```python
from build123d import *

# Parameters (mm, degrees)
EXTRUDE_2_DEPTH     = 120
SKETCH_3_W          = 40
SKETCH_3_H          = 20.78460969
EXTRUDE_3_DEPTH     = 2
SKETCH_4_W          = 17.320508076
SKETCH_4_H          = 20.78460969
EXTRUDE_4_DEPTH     = 30
SKETCH_5_W          = 40
SKETCH_5_H          = 17.320508076
EXTRUDE_5_DEPTH     = 80
SKETCH_6_R          = 1.75
CUT_EXTRUDE_1_DEPTH = 234.786227139
SKETCH_7_R          = 3.25
CUT_EXTRUDE_2_DEPTH = 3.5
SKETCH_8_W          = 40
SKETCH_8_H          = 20
CUT_EXTRUDE_3_DEPTH = 1
SKETCH_10_W         = 40
SKETCH_10_H         = 20
CUT_EXTRUDE_4_DEPTH = 1
SKETCH_11_W         = 20
SKETCH_11_H         = 40
CUT_EXTRUDE_5_DEPTH = 1


with BuildPart() as part:
    # ｽｹｯﾁ2 → ﾎﾞｽ - 押し出し2 (new body)
    with BuildSketch(Plane(origin=(0, 0, 0), x_dir=(-1, 0, 0), z_dir=(0, 0, -1))):
        Polygon((12, -10.392304845), (0, 10.392304845), (-12, -10.392304845), align=None)
    extrude(amount=EXTRUDE_2_DEPTH)

    # ｽｹｯﾁ3 → ﾎﾞｽ - 押し出し3 (add)
    with BuildSketch(Plane(origin=(0, 0, -120), x_dir=(-1, 0, 0), z_dir=(0, 0, -1))):
        Rectangle(SKETCH_3_W, SKETCH_3_H)
    extrude(amount=EXTRUDE_3_DEPTH)

    # ｽｹｯﾁ4 → ﾎﾞｽ - 押し出し4 (add)
    with BuildSketch(Plane(origin=(0, 0, -122), x_dir=(-1, 0, 0), z_dir=(0, 0, -1))):
        Rectangle(SKETCH_4_W, SKETCH_4_H)
    extrude(amount=EXTRUDE_4_DEPTH)

    # ｽｹｯﾁ5 → ﾎﾞｽ - 押し出し5 (add)
    with BuildSketch(Plane(origin=(0, 0, -152), x_dir=(-1, 0, 0), z_dir=(0, 0, -1))):
        Rectangle(SKETCH_5_W, SKETCH_5_H)
    extrude(amount=EXTRUDE_5_DEPTH)

    # ｽｹｯﾁ6 → ｶｯﾄ - 押し出し1 (cut, through all)
    with BuildSketch(Plane(origin=(0, 10.392304845, 0), x_dir=(1, 0, 0), z_dir=(0, 1, 0))):
        with Locations(Location((-10, 162, 0), (0, 0, 270))):
            Circle(SKETCH_6_R)
        with Locations(Location((10, 162, 0), (0, 0, 270))):
            Circle(SKETCH_6_R)
        with Locations(Location((-10, 222, 0), (0, 0, 270))):
            Circle(SKETCH_6_R)
        with Locations(Location((10, 222, 0), (0, 0, 270))):
            Circle(SKETCH_6_R)
    extrude(amount=-CUT_EXTRUDE_1_DEPTH, mode=Mode.SUBTRACT)

    # ｽｹｯﾁ7 → ｶｯﾄ - 押し出し2 (cut)
    with BuildSketch(Plane(origin=(0, 10.392304845, 0), x_dir=(1, 0, 0), z_dir=(0, 1, 0))):
        with Locations(Location((-10, 162, 0), (0, 0, 270))):
            Circle(SKETCH_7_R)
        with Locations(Location((-10, 222, 0), (0, 0, 270))):
            Circle(SKETCH_7_R)
        with Locations(Location((10, 222, 0), (0, 0, 270))):
            Circle(SKETCH_7_R)
        with Locations(Location((10, 162, 0), (0, 0, 270))):
            Circle(SKETCH_7_R)
    extrude(amount=-CUT_EXTRUDE_2_DEPTH, mode=Mode.SUBTRACT)

    # ｽｹｯﾁ8 → ｶｯﾄ - 押し出し3 (cut)
    with BuildSketch(Plane(origin=(-4.5, 2.598076211, 0), x_dir=(0, 0, 1), z_dir=(-0.8660254037844386, 0.5000000000000001, 0))):
        with Locations((-95, -3)):
            Rectangle(SKETCH_8_W, SKETCH_8_H)
        with Locations((-25, -3)):
            Rectangle(SKETCH_8_W, SKETCH_8_H)
    extrude(amount=-CUT_EXTRUDE_3_DEPTH, mode=Mode.SUBTRACT)

    # ｽｹｯﾁ10 → ｶｯﾄ - 押し出し4 (cut)
    with BuildSketch(Plane(origin=(4.5, 2.598076211, 0), x_dir=(0, 0, -1), z_dir=(0.8660254037844387, 0.5000000000000001, 0))):
        with Locations((25, -3)):
            Rectangle(SKETCH_10_W, SKETCH_10_H)
        with Locations((95, -3)):
            Rectangle(SKETCH_10_W, SKETCH_10_H)
    extrude(amount=-CUT_EXTRUDE_4_DEPTH, mode=Mode.SUBTRACT)

    # ｽｹｯﾁ11 → ｶｯﾄ - 押し出し5 (cut)
    with BuildSketch(Plane(origin=(0, -10.392304845, 0), x_dir=(-1, 0, 0), z_dir=(0, -1, 0))):
        with Locations((0, 25)):
            Rectangle(SKETCH_11_W, SKETCH_11_H)
        with Locations((0, 95)):
            Rectangle(SKETCH_11_W, SKETCH_11_H)
    extrude(amount=-CUT_EXTRUDE_5_DEPTH, mode=Mode.SUBTRACT)


solid = part.part
```
For this review, take the finished solid that the model builds, in its own axes (mm). A direction names the side the tool comes from. Round coordinates to 2 decimals unless told otherwise and drop trailing zeros. Write each loop counter-clockwise with the first axis right and the second up, starting at its lowest first coordinate (ties: lowest second). Pieces come first, ordered by that corner, then holes. Notation, with made-up numbers: (87, 28) -> (119, 28) arc R12 ccw to (119, 42) -> close; hole circle Ø6 at (75, -34.5). An arc over 180 degrees is marked (long way). One line per question, with ' | ' between items. Start each with the question number.
(1) Add section C-C, the plane y = -1.25. Give the number of separate pieces and of enclosed holes in the cut face, plus the area to 3 significant figures.
(2) For line 1 along X through (y, z) = (8.05, -222); line 2 along Z through (x, y) = (-11.5, 5); line 3 along Z through (x, y) = (-7.5, -3), list the stretches that pass through material, from the lowest coordinate up. Write a range as from..to.
(3) Add section D-D, the plane z = -206.5. Write out the cut boundary in (x, y), plus the area to 3 significant figures.
(4) Insertion check: P1, Ø4, axis at x = 3, z = -176.5, coming from the -Y side; P2, Ø0.5, axis at y = -10, z = -31.5, coming from the +X side; P3, Ø3, axis at x = 9, z = -160.5, coming from the +Y side. Each pin has a flat end and moves straight along its axis. Give the tip position at first contact, or say it passes through.
(5) Add section A-A, the plane x = 17. Write out the cut boundary in (y, z), plus the area to 3 significant figures.
(6) Add section B-B, the plane z = -17.5. Write out the cut boundary in (x, y), plus the area to 3 significant figures.
(7) Mouldability with a two-part tool opening along X and no side actions: class faces 1 (the face through (10.5, -10.392, -81.3)), 2 (the face through (-9.02, 7.79, -158.9)), 3 (the face through (6, 0, -59)) as released by +X, released by -X, zero draft, split by the parting line, or undercut.
(8) Tool access review of faces 4 (the face through (12, 2, -120)), 5 (the face through (0, -8.66, -191)), 6 (the face through (-14, 0, -122)): name each direction out of +Z, -Z, +X, -X, +Y, -Y from which nothing blocks a thin tool from reaching the whole face with its end or side.
Answer list:
1) separate pieces: 1 | enclosed holes: 4 | area: 5,190 mm²
2) line 1: -20..-13.25, -6.75..6.75, 13.25..20 | line 2: -232..-222.9, -221.1..-162.9, -161.1..-152, -122..-120 | line 3: -232..-115, -75..-45, -5..0
3) outline: (-20, -8.66) -> (20, -8.66) -> (20, 8.66) -> (-20, 8.66) -> close | area: 693 mm²
4) P1: y = -8.66 | P2: x = 11.92 | P3: y = 8.66
5) outline: (-10.39, -122) -> (10.39, -122) -> (10.39, -120) -> (-10.39, -120) -> close; (-8.66, -232) -> (8.66, -232) -> (8.66, -152) -> (-8.66, -152) -> close | area: 1,430 mm²
6) outline: (-12, -10.39) -> (-10, -10.39) -> (-10, -9.39) -> (10, -9.39) -> (10, -10.39) -> (12, -10.39) -> (11, -8.66) -> (10.13, -9.16) -> (0.13, 8.16) -> (1, 8.66) -> (0, 10.39) -> (-1, 8.66) -> (-0.13, 8.16) -> (-10.13, -9.16) -> (-11, -8.66) -> close | area: 189 mm²
7) face 1: zero draft | face 2: undercut | face 3: released by +X
8) face 4: +Z, +X, +Y | face 5: -Z, +X, -X, -Y | face 6: -X, +Y, -Y
